from build123d import *

# Parameters (mm, degrees)
BOSS_EXTRUDE2_DEPTH            = 5
M6_CLEARANCE_HOLE2_D           = 6.6
M6_CLEARANCE_HOLE2_CSINK_D     = 6.65
M6_CLEARANCE_HOLE2_CSINK_ANGLE = 90


with BuildPart() as part:
    # Sketch1 → Boss-Extrude2 (new body)
    with BuildSketch(Plane.XY):
        Polygon((-37.5, 20.889), (-101.6, 20.889), (-101.6, 173.289), (101.6, 173.289), (101.6, 20.889), (37.5, 20.889), (37.5, -20.889), (-37.5, -20.889), align=None)
    extrude(amount=BOSS_EXTRUDE2_DEPTH)

    # M6 Clearance Hole2 (through all)
    with Locations(Plane.XY.offset(5)):
        with Locations((-22.5, 5.889), (22.5, 5.889)):
            CounterSinkHole(M6_CLEARANCE_HOLE2_D / 2, M6_CLEARANCE_HOLE2_CSINK_D / 2, counter_sink_angle=M6_CLEARANCE_HOLE2_CSINK_ANGLE)


solid = part.part
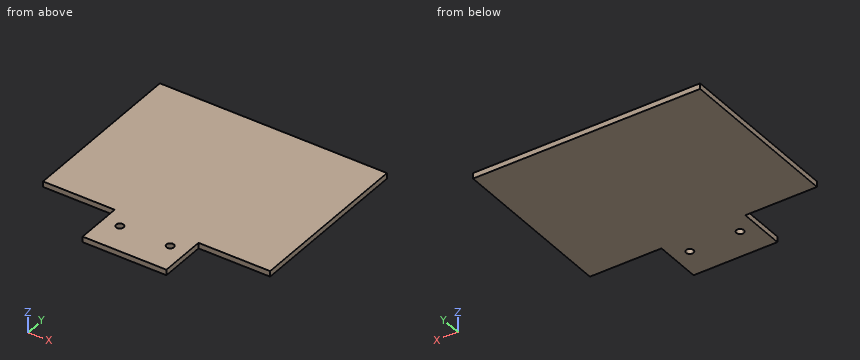
Verification items for the finished model (mm, model axes). Coordinates: 2 decimals unless noted, no trailing zeros. Order: outer loops, then holes, each group sorted by start corner. A loop starts at its lowest first (then second) coordinate and runs counter-clockwise, first axis right, second up. Notation, with made-up numbers: M 10.5,73.25 L 63.5,73.25 A12 cw 63.5,80.25 Z; hole C 79,-36 d4. An arc over 180 degrees is marked long. One line per item, written item: value. Start each with the question number.
Item 1: Sectioned sample at D-D on x = -63.5. Record the cut outline in (y, z), then the cut area to 3 significant figures.
Item 2: Sectioned sample at A-A on x = 22.5. Record the cut outline in (y, z) (3 decimals), then the cut area to 3 significant figures.
Item 3: Depth check by flat-ended pin: P1, Ø1.5, axis at x = 63, z = 1.5, coming from the -Y side; P2, Ø1.5, axis at y = 1, z = 2.5, coming from the +X side; P3, Ø2.5, axis at y = -4, z = 2, coming from the -X side. Enter the tip coordinate at first touch or a pass-through.
Item 4: Sectioned sample at B-B on z = 1.4. Record the cut outline in (x, y).
Item 5: Thickness scan on probe 1 along Y at (x, z) = (-22.5, 2.75); probe 2 along Y at (x, z) = (24.5, 1.6); probe 3 along Y at (x, z) = (72, 1). Record the ranges inside material, lowest first.
Item 6: Sectioned sample at C-C on y = -2. Record the cut outline in (x, z).
Calculated:
1. outline: M 20.89,0 L 173.29,0 L 173.29,5 L 20.89,5 Z
1. area: 762 mm^2
2. outline: M -20.889,0 L 2.589,0 L 2.589,4.975 L 2.564,5 L -20.889,5 Z; M 9.189,0 L 173.289,0 L 173.289,5 L 9.214,5 L 9.189,4.975 Z
2. area: 938 mm^2
3. P1: y = 20.89
3. P2: x = 37.5
3. P3: x = -37.5
4. outline: M -101.6,20.89 L -37.5,20.89 L -37.5,-20.89 L 37.5,-20.89 L 37.5,20.89 L 101.6,20.89 L 101.6,173.29 L -101.6,173.29 Z; hole C -22.5,5.89 d6.6; hole C 22.5,5.89 d6.6
5. probe 1: -20.89 to 2.59, 9.19 to 173.29
5. probe 2: -20.89 to 3.26, 8.51 to 173.29
5. probe 3: 20.89 to 173.29
6. outline: M -37.5,0 L 37.5,0 L 37.5,5 L -37.5,5 Z
